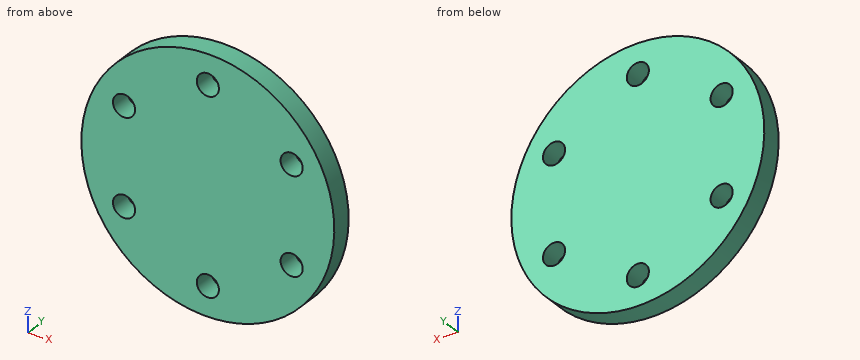
from build123d import *

# Parameters (mm, degrees)
SKETCH1_R           = 60.088817471
BOSS_EXTRUDE1_DEPTH = 10
SKETCH2_R           = 5.255125099
CUT_EXTRUDE1_DEPTH  = 10
CIRPATTERN1_COUNT   = 6


with BuildPart() as part:
    # Sketch1 → Boss-Extrude1 (new body)
    with BuildSketch(Plane(origin=(0, 0, 0), x_dir=(1, 0, 0), z_dir=(0, 1, 0))):
        with Locations(Location((0, 0, 0), (0, 0, 270))):
            Circle(SKETCH1_R)
    extrude(amount=BOSS_EXTRUDE1_DEPTH)

    # Sketch2 → Cut-Extrude1 (cut)
    with BuildSketch(Plane(origin=(0, 0, 0), x_dir=(1, 0, 0), z_dir=(0, 1, 0))):
        with Locations(Location((0, 45.976959249, 0), (0, 0, 270))):
            Circle(SKETCH2_R)
    cut_extrude1 = extrude(amount=CUT_EXTRUDE1_DEPTH, mode=Mode.SUBTRACT)

    # CirPattern1: Cut-Extrude1 ×6 about axis
    cirpattern1_axis = Axis((0, 0, 0), (0, 1, 0))
    for i in range(1, CIRPATTERN1_COUNT):
        add(cut_extrude1.rotate(cirpattern1_axis, i * 360 / CIRPATTERN1_COUNT), mode=Mode.SUBTRACT)


solid = part.part
Could you check a few things on this model? Use its own coordinates, in mm. Give positions to 0.01 mm unless a question says otherwise; leave off trailing zeros. Order: outer loops, then holes, each group sorted by start corner. A loop starts at its lowest first (then second) coordinate and runs counter-clockwise, first axis right, second up.
Item 1: If we section it at A-A, the plane x = 0: Write out the boundary of the cut face in (y, z).
Item 2: I'm going to push flat-ended pins straight in: pin 1 (6 mm diameter, centred on x = -47.5, y = 1.5, fed in from -Z); pin 2 (1.5 mm diameter, centred on x = -35, y = 4, fed in from +Z); pin 3 (1 mm diameter, centred on x = 18, y = 3.5, fed in from +Z). Where does each tip first touch, or does it pass through?
Item 3: If we section it at B-B, the plane y = 8: Write out the boundary of the cut face in (x, z), plus the area to 3 significant figures.
Item 4: I need wall thicknesses on line 1 (Z direction, x = -2.5, y = 1); line 2 (X direction, y = 8.75, z = -25); line 3 (X direction, y = 6.75, z = -0.5). Which ranges of each line are inside material? Lowest first, please.
Item 5: If we section it at C-C, the plane z = 42.5: Write out the boundary of the cut face in (x, y).
Item 6: If we section it at D-D, the plane x = -42: Write out the boundary of the cut face in (y, z), plus the area to 3 significant figures.
Values:
1. outline: (0, -60.09) - (10, -60.09) - (10, -51.23) - (0, -51.23) - close; (0, -40.72) - (10, -40.72) - (10, 40.72) - (0, 40.72) - close; (0, 51.23) - (10, 51.23) - (10, 60.09) - (0, 60.09) - close
2. pin 1: stops at z = -40.38
2. pin 2: stops at z = 49.37
2. pin 3: stops at z = 57.48
3. outline: circle Ø120.18 at (0, 0); hole circle Ø10.51 at (-39.82, -22.99); hole circle Ø10.51 at (-39.82, 22.99); hole circle Ø10.51 at (0, -45.98); hole circle Ø10.51 at (0, 45.98); hole circle Ø10.51 at (39.82, -22.99); hole circle Ø10.51 at (39.82, 22.99)
3. area: 10,800 mm2
4. line 1: z = -60.04 to -50.6, -41.35 to 41.35, 50.6 to 60.04
4. line 2: x = -54.64 to -44.67, -34.96 to 34.96, 44.67 to 54.64
4. line 3: x = -60.09 to 60.09
5. outline: (-42.48, 0) - (-3.94, 0) - (-3.94, 10) - (-42.48, 10) - close; (3.94, 0) - (42.48, 0) - (42.48, 10) - (3.94, 10) - close
6. outline: (0, -42.97) - (10, -42.97) - (10, -27.77) - (0, -27.77) - close; (0, -18.21) - (10, -18.21) - (10, 18.21) - (0, 18.21) - close; (0, 27.77) - (10, 27.77) - (10, 42.97) - (0, 42.97) - close
6. area: 668 mm2
